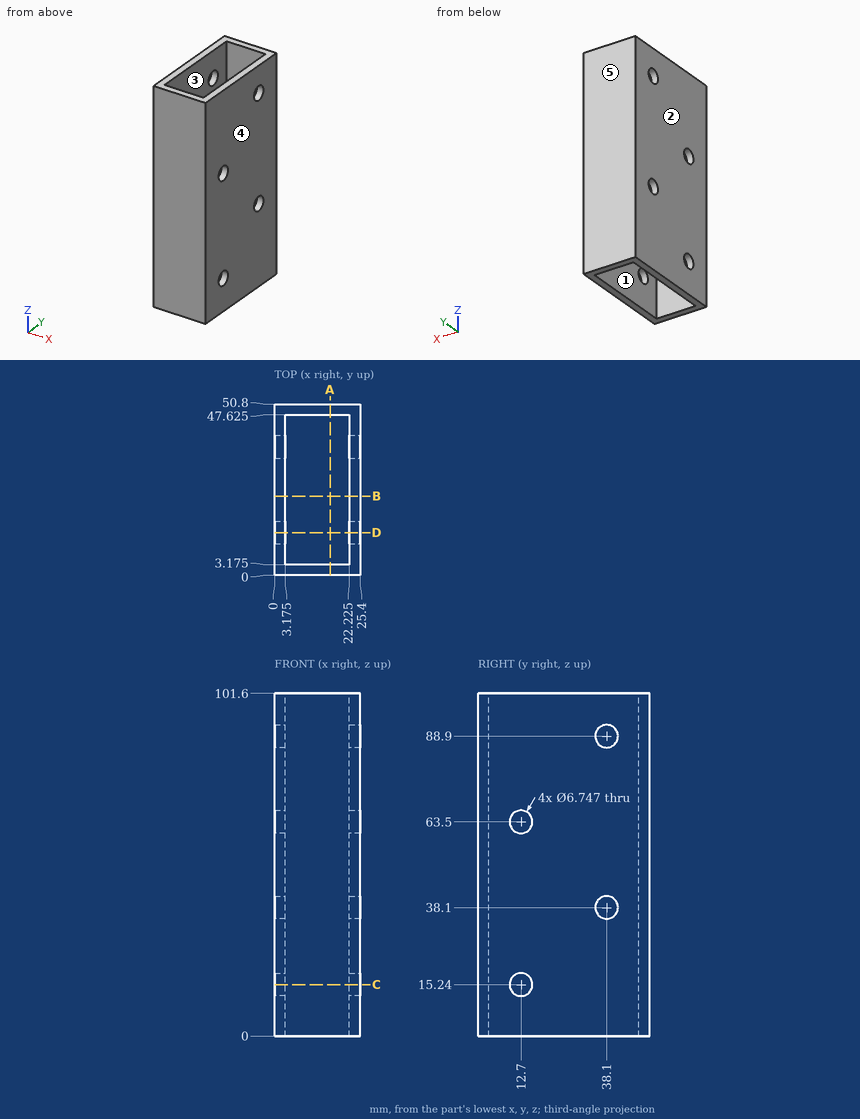
Geometry check sheet. Reference: drawing and pictorial views, mm from the part's lowest x, y, z. A direction names the side the tool comes from. Round coordinates to 2 decimals unless told otherwise and drop trailing zeros. Loops run counter-clockwise (first coordinate to the right, second up) from the corner with the lowest first, then second, coordinate; pieces in that order, holes last. Notation, with made-up numbers: (85.5, 20.25) -> (117.5, 20.25) arc R15 cw to (117.5, 44.25) -> close; hole circle Ø5 at (42, -11.5). An arc over 180 degrees is marked (long way). Answer as a JSON object with one key per item and string values. Group by question number.
Item 1: Cross-section at B-B, the plane y = 23.5. Record the cut outline in (x, z) (3 decimals).
Item 2: Thickness scan on line 1 along Y through (x, z) = (12, 88) (3 decimals); line 2 along X through (y, z) = (45, 93.5) (3 decimals); line 3 along Y through (x, z) = (1.85, 63.5). Record the ranges inside material, lowest first.
Item 3: Cross-section at C-C, the plane z = 15.24. Record the cut outline in (x, y) (1 decimal).
Item 4: Cross-section at A-A, the plane x = 16.5. Record the cut outline in (y, z) (3 decimals).
Item 5: Set-up check for the marked faces 1 and 2: record each of +Z, -Z, +X, -X, +Y, -Y from which the full face is reachable in a straight line by a thin tool's end or side.
Item 6: Release check for a two-part mould opening along X. For the marked faces 3, 4 and 5 record: pulls with the +X half, pulls with the -X half, needs draft (parallel to the pull), parting line crosses it, or undercut.
Item 7: Cross-section at D-D, the plane y = 12.7. Record the cut outline in (x, z) (1 decimal).
Determined:
{
 "1": {"outline": "(0, 0) -> (3.175, 0) -> (3.175, 101.6) -> (0, 101.6) -> close; (22.225, 0) -> (25.4, 0) -> (25.4, 101.6) -> (22.225, 101.6) -> close"},
 "2": {"line 1": "y = 0 to 3.175, 47.625 to 50.8", "line 2": "x = 0 to 3.175, 22.225 to 25.4", "line 3": "y = 0 to 9.33, 16.07 to 50.8"},
 "3": {"outline": "(0, 0) -> (25.4, 0) -> (25.4, 9.3) -> (22.2, 9.3) -> (22.2, 3.2) -> (3.2, 3.2) -> (3.2, 9.3) -> (0, 9.3) -> close; (0, 16.1) -> (3.2, 16.1) -> (3.2, 47.6) -> (22.2, 47.6) -> (22.2, 16.1) -> (25.4, 16.1) -> (25.4, 50.8) -> (0, 50.8) -> close"},
 "4": {"outline": "(0, 0) -> (3.175, 0) -> (3.175, 101.6) -> (0, 101.6) -> close; (47.625, 0) -> (50.8, 0) -> (50.8, 101.6) -> (47.625, 101.6) -> close"},
 "5": {"face 1": "+Z, -Z", "face 2": "+Z, -Z, -X, +Y, -Y"},
 "6": {"face 3": "undercut", "face 4": "pulls with the +X half", "face 5": "needs draft"},
 "7": {"outline": "(0, 0) -> (3.2, 0) -> (3.2, 11.9) -> (0, 11.9) -> close; (0, 18.6) -> (3.2, 18.6) -> (3.2, 60.1) -> (0, 60.1) -> close; (0, 66.9) -> (3.2, 66.9) -> (3.2, 101.6) -> (0, 101.6) -> close; (22.2, 0) -> (25.4, 0) -> (25.4, 11.9) -> (22.2, 11.9) -> close; (22.2, 18.6) -> (25.4, 18.6) -> (25.4, 60.1) -> (22.2, 60.1) -> close; (22.2, 66.9) -> (25.4, 66.9) -> (25.4, 101.6) -> (22.2, 101.6) -> close"}
}
